Source: CAD feature listing. Evaluate the final solid. Frame: model axes, mm. Give positions to 0.01 mm unless a question says otherwise; leave off trailing zeros. Write each loop counter-clockwise with the first axis right and the second up, starting at its lowest first coordinate (ties: lowest second). Pieces come first, ordered by that corner, then holes. Notation, with made-up numbers: (45.5, 86) -> (92.5, 86) arc R16 ccw to (92.5, 109) -> close; hole circle Ø9 at (-28, 24). An arc over 180 degrees is marked (long way). Write item = value, one per line.
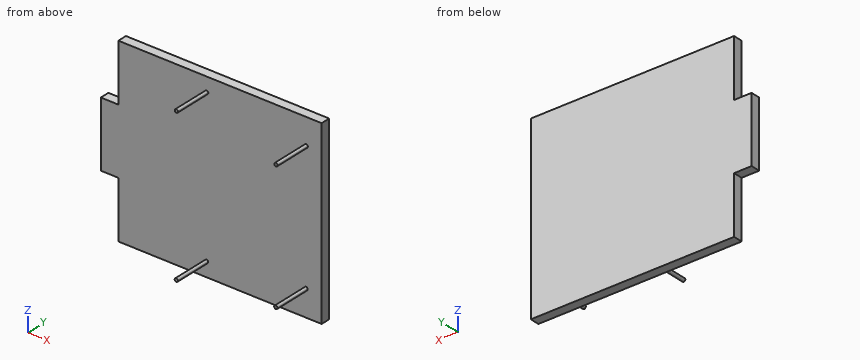
from build123d import *

# Parameters (mm, degrees)
BOSS_EXTRUDE1_DEPTH = 10
SKETCH2_R           = 1.75
BOSS_EXTRUDE2_DEPTH = 40


with BuildPart() as part:
    # Sketch1 → Boss-Extrude1 (new body)
    with BuildSketch(Plane(origin=(0, 0, 0), x_dir=(1, 0, 0), z_dir=(0, 1, 0))):
        Polygon((196.990512748, 28.023652023), (414.922512748, 28.023652023), (414.922512748, -165.016347977), (196.990512748, -165.016347977), (196.990512748, -103.548347977), (178.194512748, -103.548347977), (178.194512748, -33.190347977), (196.990512748, -33.190347977), align=None)
    extrude(amount=BOSS_EXTRUDE1_DEPTH)

    # Sketch2 → Boss-Extrude2 (add)
    with BuildSketch(Plane.XZ):
        with Locations((291.700512748, 149.842465897)):
            Circle(SKETCH2_R)
        with Locations((398.380512748, 137.085232309)):
            Circle(SKETCH2_R)
        with Locations((398.306929068, -0.074747953)):
            Circle(SKETCH2_R)
        with Locations((291.61330246, -12.71751071)):
            Circle(SKETCH2_R)
    extrude(amount=BOSS_EXTRUDE2_DEPTH)


solid = part.part
1) Cut plane B-B (z = 84.5). Return the cut outline in (x, y), then the cut area to 3 significant figures.
Computed:
outline = (178.19, 0) -> (414.92, 0) -> (414.92, 10) -> (178.19, 10) -> close
area = 2,370 mm²
2) Material intervals for L1, parallel to Y at x = 326.5, z = 90.5; L2, parallel to X at y = 5.5, z = 30, sorted ascending.
Computed:
L1 = 0 to 10
L2 = 196.99 to 414.92
3) Contact query for flat-ended pins moving along their axis: pin 1 (1 mm diameter, centred on x = 264, z = 80.5, fed in from -Y); pin 2 (3 mm diameter, centred on x = 184, y = 5, fed in from -Z); pin 3 (8 mm diameter, centred on y = 6, z = 12.5, fed in from -X). Output: stop coordinate, or through.
Computed:
pin_1 = 0
pin_2 = 33.19
pin_3 = 196.99
4) Cut plane D-D (y = -35.5). Return the cut outline in (x, z).
Computed:
outline = circle Ø3.5 at (291.61, -12.72); circle Ø3.5 at (291.7, 149.84); circle Ø3.5 at (398.31, -0.07); circle Ø3.5 at (398.38, 137.09)
5) Cut plane C-C (x = 244). Return the cut outline in (y, z), then the cut area to 3 significant figures.
Computed:
outline = (0, -28.02) -> (10, -28.02) -> (10, 165.02) -> (0, 165.02) -> close
area = 1,930 mm²
6) Cut plane A-A (y = 4). Return the cut outline in (x, z).
Computed:
outline = (178.19, 33.19) -> (196.99, 33.19) -> (196.99, -28.02) -> (414.92, -28.02) -> (414.92, 165.02) -> (196.99, 165.02) -> (196.99, 103.55) -> (178.19, 103.55) -> close
